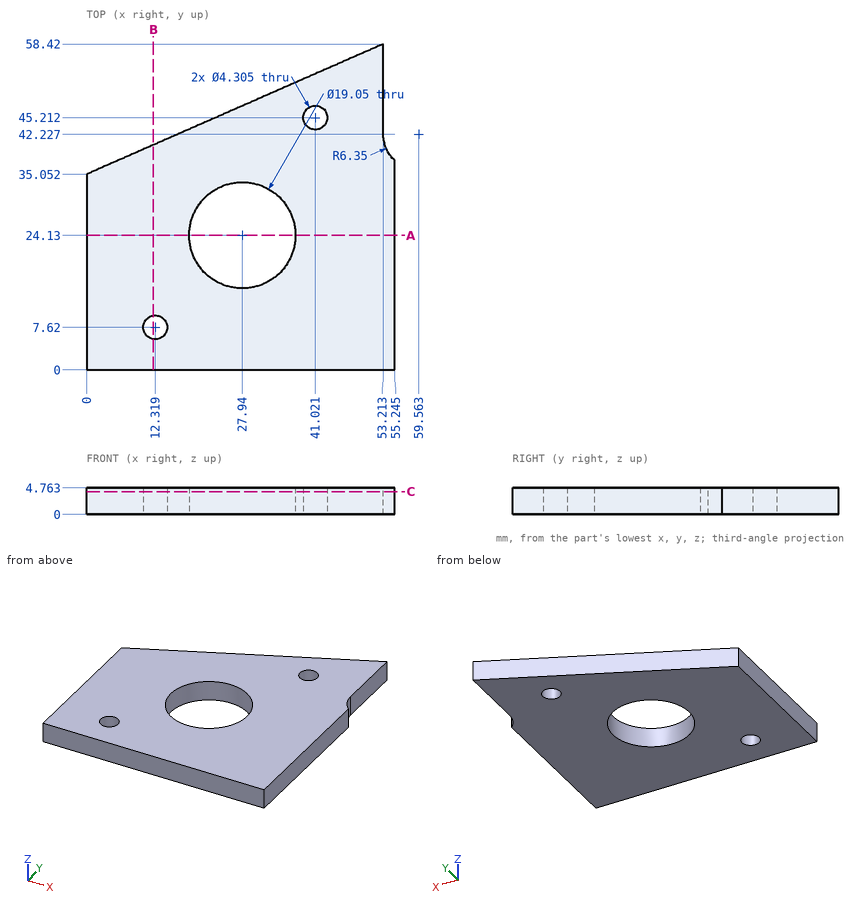
For this review, use the dimensioned drawing (mm, ordinates from the lowest corner) and the shaded views. Round coordinates to 2 decimals unless told otherwise and drop trailing zeros. Loops run counter-clockwise (first coordinate to the right, second up) from the corner with the lowest first, then second, coordinate; pieces in that order, holes last. Notation, with made-up numbers: M -29,-1.75 L 10,-1.75 A25 cw 10,34.25 Z; hole C -36.5,38 d7. An arc over 180 degrees is marked long. Answer as CSV lines item,"result".
1. We need section A-A (y = 24.13). Give the boundary of the cut face in (x, z) (1 decimal).
Outcome:
outline,"M 0,0 L 18.4,0 L 18.4,4.8 L 0,4.8 Z; M 37.5,0 L 55.2,0 L 55.2,4.8 L 37.5,4.8 Z"
2. We need section C-C (z = 4.1). Count the separate pieces of the cut face and the enclosed holes in it, plus the area to 3 significant figures.
Outcome:
separate pieces,"1"
enclosed holes,"3"
area,"2,250 mm2"
3. We need section B-B (x = 12). Give the boundary of the cut face in (y, z), plus the area to 3 significant figures.
Outcome:
outline,"M 0,0 L 5.49,0 L 5.49,4.76 L 0,4.76 Z; M 9.75,0 L 40.32,0 L 40.32,4.76 L 9.75,4.76 Z"
area,"172 mm2"
4. To check wall thickness, follow L1, parallel to Y at x = 27.94, z = 2.85 (1 decimal); L2, parallel to X at y = 17, z = 3.65 (1 decimal); L3, parallel to X at y = 25, z = 1.3 (1 decimal). State the ranges of each line that lie inside material, in increasing order. Write a range as [from, to].
Outcome:
L1,"y = [0, 14.6], [33.7, 47.3]"
L2,"x = [0, 21.6], [34.3, 55.2]"
L3,"x = [0, 18.5], [37.4, 55.2]"
5. Insertion check: pin 1 Ø1.5 at (y, z) = (38.5, 1.5) entering from -X (1 decimal); pin 2 Ø1.4 at (y, z) = (52.5, 3) entering from +X; pin 3 Ø15 at (x, y) = (27.94, 24.13) entering from +Z. Each pin has a flat end and moves straight along its axis. Give the tip position at first contact, or say it passes through.
Outcome:
pin 1,"stops at x = 6.1"
pin 2,"stops at x = 53.21"
pin 3,"passes through"
